The model under review builds one solid part; all positions refer to its coordinate system, in mm. Face numbers are marked on the shaded views. A direction names the side the tool comes from. Give positions to 0.01 mm unless a question says otherwise; leave off trailing zeros. Loops run counter-clockwise (first coordinate to the right, second up) from the corner with the lowest first, then second, coordinate; pieces in that order, holes last. Notation, with made-up numbers: (24.5, 36) - (32.5, 36) arc R15 ccw to (32.5, 52) - close; hole circle Ø6 at (44.25, 31.5). An arc over 180 degrees is marked (long way). Return JSON: item names as keys, results as strings. Group by question number.
```python
from build123d import *

# Parameters (mm, degrees)
BOSS_EXTRUDE2_DEPTH = 65
CUT_EXTRUDE1_DEPTH  = 54
FILLET1_R           = 5
FILLET2_R           = 1
BOSS_EXTRUDE3_DEPTH = 2.5
FILLET4_R           = 2
FILLET5_R           = 1
SKETCH4_R           = 3
SKETCH4_R_2         = 2.5
BOSS_EXTRUDE8_DEPTH = 1.75


with BuildPart() as part:
    # Sketch1 → Boss-Extrude2 (new, symmetric)
    with BuildSketch(Plane.XY):
        with BuildLine():
            Line((-12, -11), (-12, 11))
            ThreePointArc((-12, 11), (0, 23), (12, 11))
            Line((12, 11), (12, -11))
            ThreePointArc((12, -11), (0, -23), (-12, -11))
        make_face()
    extrude(amount=BOSS_EXTRUDE2_DEPTH, both=True)

    # Sketch2 → Cut-Extrude1 (cut, symmetric)
    with BuildSketch(Plane.XY):
        with BuildLine():
            Line((15, 11), (15, -11))
            ThreePointArc((15, -11), (0, -26), (-15, -11))
            Line((-15, -11), (-15, 11))
            ThreePointArc((-15, 11), (0, 26), (15, 11))
        make_face()
        with BuildLine():
            Line((-11.3, 11), (-11.3, -11))
            ThreePointArc((-11.3, -11), (0, -22.3), (11.3, -11))
            Line((11.3, -11), (11.3, 11))
            ThreePointArc((11.3, 11), (0, 22.3), (-11.3, 11))
        make_face(mode=Mode.SUBTRACT)
    extrude(amount=CUT_EXTRUDE1_DEPTH, both=True, mode=Mode.SUBTRACT)

    # Fillet1
    # the kernel refuses this fillet: 5 mm, written as the material it adds along each edge
    with BuildSketch(Plane(origin=(0, 11, -54), x_dir=(1, 0, 0), z_dir=(0, -1, 0))) as fillet1_piece_1:
        with BuildLine():
            CenterArc((16.3, 2.551470164), FILLET1_R, 180, 30.683417109)
            Line((11.3, 2.551470164), (11.2, 2.551470164))
            Line((11.2, 2.551470164), (11.2, 0))
            Line((11.2, 0), (11.3, -0.1))
            ThreePointArc((11.3, -0.1), (11.65, -0.1), (11.914, -0.051029403))
            Line((11.914, -0.051029403), (12, 0))
        make_face()
    revolve(axis=Axis((0, 11, -54), (0, 0, 1)), revolution_arc=180)
    with BuildSketch(Plane(origin=(-11.3, 11, -54), x_dir=(-1, 0, 0), z_dir=(0, -1, 0)), Plane(origin=(11.3, -11, -54), x_dir=(1, 0, 0), z_dir=(0, 1, 0))) as fillet1_piece_2:
        with BuildLine():
            CenterArc((5, -2.551470164), FILLET1_R, 149.316582891, 30.683417109)
            Line((0, -2.551470164), (-0.1, -2.551470164))
            Line((-0.1, -2.551470164), (-0.1, 0))
            Line((-0.1, 0), (0, 0.1))
            ThreePointArc((0, 0.1), (0.35, 0.1), (0.614, 0.051029403))
            Line((0.614, 0.051029403), (0.7, 0))
        make_face()
    extrude(amount=22)
    with BuildSketch(Plane(origin=(0, -11, -54), x_dir=(-1, 0, 0), z_dir=(0, 1, 0))) as fillet1_piece_3:
        with BuildLine():
            CenterArc((16.3, 2.551470164), FILLET1_R, 180, 30.683417109)
            Line((11.3, 2.551470164), (11.2, 2.551470164))
            Line((11.2, 2.551470164), (11.2, 0))
            Line((11.2, 0), (11.3, -0.1))
            ThreePointArc((11.3, -0.1), (11.65, -0.1), (11.914, -0.051029403))
            Line((11.914, -0.051029403), (12, 0))
        make_face()
    revolve(axis=Axis((0, -11, -54), (0, 0, 1)), revolution_arc=180)
    with BuildSketch(Plane(origin=(0, 11, 54), x_dir=(1, 0, 0), z_dir=(0, -1, 0))) as fillet1_piece_4:
        with BuildLine():
            CenterArc((16.3, -2.551470164), FILLET1_R, 149.316582891, 30.683417109)
            Line((12, 0), (11.914, 0.051029403))
            ThreePointArc((11.914, 0.051029403), (11.65, 0.1), (11.3, 0.1))
            Line((11.3, 0.1), (11.2, 0))
            Line((11.2, 0), (11.2, -2.551470164))
            Line((11.2, -2.551470164), (11.3, -2.551470164))
        make_face()
    revolve(axis=Axis((0, 11, 54), (0, 0, 1)), revolution_arc=180)
    with BuildSketch(Plane(origin=(11.3, -11, 54), x_dir=(0, 0, -1), z_dir=(0, 1, 0)), Plane(origin=(-11.3, 11, 54), x_dir=(0, 0, -1), z_dir=(0, -1, 0))) as fillet1_piece_5:
        with BuildLine():
            CenterArc((2.551470164, -5), FILLET1_R, 90, 30.683417109)
            Line((0, -0.7), (-0.051029403, -0.614))
            ThreePointArc((-0.051029403, -0.614), (-0.1, -0.35), (-0.1, 0))
            Line((-0.1, 0), (0, 0.1))
            Line((0, 0.1), (2.551470164, 0.1))
            Line((2.551470164, 0.1), (2.551470164, 0))
        make_face()
    extrude(amount=22)
    with BuildSketch(Plane(origin=(0, -11, 54), x_dir=(-1, 0, 0), z_dir=(0, 1, 0))) as fillet1_piece_6:
        with BuildLine():
            CenterArc((16.3, -2.551470164), FILLET1_R, 149.316582891, 30.683417109)
            Line((12, 0), (11.914, 0.051029403))
            ThreePointArc((11.914, 0.051029403), (11.65, 0.1), (11.3, 0.1))
            Line((11.3, 0.1), (11.2, 0))
            Line((11.2, 0), (11.2, -2.551470164))
            Line((11.2, -2.551470164), (11.3, -2.551470164))
        make_face()
    revolve(axis=Axis((0, -11, 54), (0, 0, 1)), revolution_arc=180)

    # Fillet2
    fillet2_edges = [part.edges().sort_by_distance(p)[0] for p in [
        (0, 23, 65),
        (-12, 0, 65),
        (0, -23, 65),
        (-12, 0, -65),
        (0, 23, -65),
        (12, 0, -65),
        (0, -23, -65),
        (12, 0, 65),
    ]]
    fillet(fillet2_edges, radius=FILLET2_R)

    # Sketch3 → Boss-Extrude3 (add)
    with BuildSketch(Plane.XY.offset(65)):
        with BuildLine():
            Line((-6.5, -11.25), (-6.5, 11.25))
            ThreePointArc((-6.5, 11.25), (0, 17.75), (6.5, 11.25))
            Line((6.5, 11.25), (6.5, -11.25))
            ThreePointArc((6.5, -11.25), (0, -17.75), (-6.5, -11.25))
        make_face()
    extrude(amount=BOSS_EXTRUDE3_DEPTH)

    # Fillet4
    fillet4_edges = [part.edges().sort_by_distance(p)[0] for p in [
        (0, -17.75, 65),
        (6.5, 0, 65),
        (0, 17.75, 65),
        (-6.5, 0, 65),
    ]]
    fillet(fillet4_edges, radius=FILLET4_R)

    # Fillet5
    # the kernel refuses this fillet: 1 mm, written as the material it takes off along each edge
    with BuildSketch(Plane(origin=(-6.5, -11.25, 67.5), x_dir=(-0.03354919019221856, 0, -0.9994370674722076), z_dir=(0, 1, 0)), Plane(origin=(6.5, 11.25, 67.5), x_dir=(0.03354919019221963, 0, -0.9994370674722076), z_dir=(0, -1, 0))) as fillet5_piece_1:
        with BuildLine():
            CenterArc((0.967295605, -0.99104977), FILLET5_R, 97.671480447, 80.405931773)
            Line((-0.032141463, -0.95750058), (-0.132085169, -0.954145661))
            Line((-0.132085169, -0.954145661), (-0.099943707, 0.003354919))
            Line((-0.099943707, 0.003354919), (0.003354919, 0.099943707))
            ThreePointArc((0.003354919, 0.099943707), (0.503073453, 0.083169112), (0.820453418, 0.099104977))
            Line((0.820453418, 0.099104977), (0.833802708, 0))
        make_face()
    extrude(amount=22.5, mode=Mode.SUBTRACT)
    with BuildSketch(Plane(origin=(0, 11.25, 67.5), x_dir=(-1, 0, 0), z_dir=(0, -1, 0))) as fillet5_piece_2:
        with BuildLine():
            CenterArc((5.541960108, 1), FILLET5_R, 270, 80.405931773)
            Line((5.541960108, 0), (5.541960108, -0.1))
            Line((5.541960108, -0.1), (6.5, -0.1))
            Line((6.5, -0.1), (6.6, 0))
            ThreePointArc((6.6, 0), (6.6, 0.5), (6.626574735, 0.816666667))
            Line((6.626574735, 0.816666667), (6.527973406, 0.833333333))
        make_face()
    revolve(axis=Axis((0, 11.25, 67.5), (0, 0, -1)), revolution_arc=180, mode=Mode.SUBTRACT)
    with BuildSketch(Plane(origin=(0, -11.25, 67.5), x_dir=(1, 0, 0), z_dir=(0, 1, 0))) as fillet5_piece_3:
        with BuildLine():
            CenterArc((5.541960108, 1), FILLET5_R, 270, 80.405931773)
            Line((5.541960108, 0), (5.541960108, -0.1))
            Line((5.541960108, -0.1), (6.5, -0.1))
            Line((6.5, -0.1), (6.6, 0))
            ThreePointArc((6.6, 0), (6.6, 0.5), (6.626574735, 0.816666667))
            Line((6.626574735, 0.816666667), (6.527973406, 0.833333333))
        make_face()
    revolve(axis=Axis((0, -11.25, 67.5), (0, 0, -1)), revolution_arc=180, mode=Mode.SUBTRACT)

    # Sketch4 → Boss-Extrude8 (add)
    # profile 1 of 2: a face of its own
    with BuildSketch(Plane.XY.offset(67.5)):
        with Locations(Location((0, 3.05, 0), (0, 0, 180))):
            Circle(SKETCH4_R)
        with Locations((0, 3.05)):
            Circle(SKETCH4_R_2, mode=Mode.SUBTRACT)
    # profile 2 of 2: a face of its own
    with BuildSketch(Plane.XY.offset(67.5)):
        with Locations(Location((0, -3.05, 0), (0, 0, 180))):
            Circle(SKETCH4_R)
        with Locations((0, -3.05)):
            Circle(SKETCH4_R_2, mode=Mode.SUBTRACT)
    extrude(amount=BOSS_EXTRUDE8_DEPTH)


solid = part.part
```
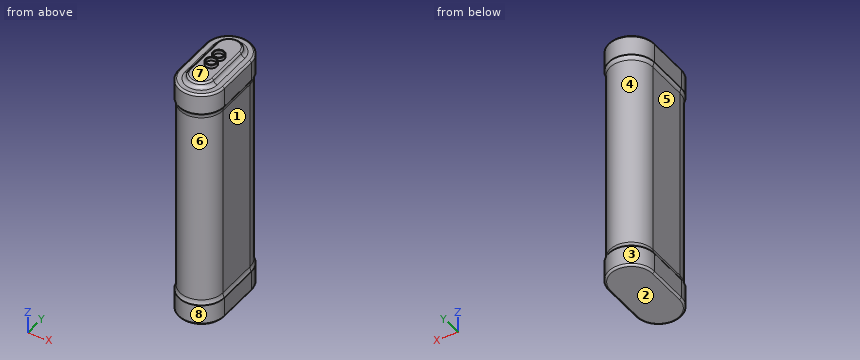
1) We need section C-C, the plane y = 8.5. Write out the cut boundary in (x, z), plus the area to 3 significant figures.
2) For pin 1 Ø5 at (x, z) = (9, -33) entering from -Y; pin 2 Ø12 at (x, z) = (2.5, -26.5) entering from +Y; pin 3 Ø6.5 at (y, z) = (2, 1.5) entering from +X, all flat-tipped, find the tip position at first contact; note any pin that passes through.
3) Draft analysis for pull direction Z (two halves, no side actions). For the marked faces 1, 2 and 3, state which applies: +Z half, -Z half, draft (parallel to the pull), parting line (faces both ways), or undercut.
4) We need section B-B, the plane z = 24.5. Write out the cut boundary in (x, y).
5) To check wall thickness, follow line 1 (X direction, y = -3, z = 68); line 2 (Z direction, x = -10.75, y = 5); line 3 (X direction, y = 3.5, z = 34). State the ranges of each line that lie inside material, in increasing order.
6) Tool access review of the marked faces 4, 5, 6, 7 and 8: name each direction out of +Z, -Z, +X, -X, +Y, -Y from which nothing blocks a thin tool from reaching the whole face with its end or side.
Findings:
{
 "1": {"outline": "(-12, -64) arc R1 ccw to (-11, -65) - (11, -65) arc R1 ccw to (12, -64) - (12, -54) arc R5 cw to (11.3, -51.45) - (11.3, 51.45) arc R5 cw to (12, 54) - (12, 64) arc R1 ccw to (11, 65) - (8.5, 65) arc R2 cw to (6.53, 66.67) arc R1 ccw to (5.54, 67.5) - (-5.54, 67.5) arc R1 ccw to (-6.53, 66.67) arc R2 cw to (-8.5, 65) - (-11, 65) arc R1 ccw to (-12, 64) - (-12, 54) arc R5 cw to (-11.3, 51.45) - (-11.3, -51.45) arc R5 cw to (-12, -54) - close", "area": "3,000 mm^2"},
 "2": {"pin 1": "stops at y = -20.24", "pin 2": "stops at y = 22.3", "pin 3": "stops at x = 11.3"},
 "3": {"face 1": "undercut", "face 2": "-Z half", "face 3": "draft"},
 "4": {"outline": "(-11.3, -11) arc R11.3 ccw to (11.3, -11) - (11.3, 11) arc R11.3 ccw to (-11.3, 11) - close"},
 "5": {"line 1": "x = -3 to -2.5, 2.5 to 3", "line 2": "z = -65 to 65", "line 3": "x = -11.3 to 11.3"},
 "6": {"face 4": "+Y", "face 5": "-X, +Y, -Y", "face 6": "-Y", "face 7": "+Z", "face 8": "+Z, -Z, -Y"}
}
